from build123d import *

# Parameters (mm, degrees)
CUT_EXTRUDE1_DEPTH = 59.523499554
SKETCH3_R          = 35
SKETCH3_R_2        = 27.5
CUT_EXTRUDE2_DEPTH = 2
CUT_EXTRUDE3_START = -2
SKETCH4_R          = 35
SKETCH4_R_2        = 27.5
CUT_EXTRUDE3_DEPTH = 2
FILLET1_R          = 10
FILLET2_R          = 10


with BuildPart() as part:
    # Sketch1 → Revolve1 (revolve)
    with BuildSketch(Plane(origin=(0, 0, 0), x_dir=(0, 0, -1), z_dir=(1, 0, 0)), mode=Mode.PRIVATE) as revolve1_sk:
        Polygon((-7.5, 40), (-4.5, 40), (-2, 34), (2, 34), (4.5, 40), (7.5, 40), (7.5, 0), (-7.5, 0), align=None)
    revolve(revolve1_sk.sketch.rotate(Axis((0, 0, 652.003718611), (0, 0, -1)), 90), axis=Axis((0, 0, 652.003718611), (0, 0, -1)))

    # Sketch2 → Cut-Extrude1 (cut, through all)
    with BuildSketch(Plane.XY.offset(7.5)):
        with BuildLine():
            Line((3.2, 15.520204103), (-2.8, 15.520204103))
            Line((-2.8, 15.520204103), (-2.8, 13.71714256))
            ThreePointArc((-2.8, 13.71714256), (-0.204757333, -13.998502578), (3.2, 13.62938003))
            Line((3.2, 13.62938003), (3.2, 15.520204103))
        make_face()
    extrude(amount=-CUT_EXTRUDE1_DEPTH, mode=Mode.SUBTRACT)

    # Sketch3 → Cut-Extrude2 (cut)
    with BuildSketch(Plane.XY.offset(7.5)):
        Circle(SKETCH3_R)
        Circle(SKETCH3_R_2, mode=Mode.SUBTRACT)
    extrude(amount=-CUT_EXTRUDE2_DEPTH, mode=Mode.SUBTRACT)

    # Sketch4 → Cut-Extrude3 (cut)
    with BuildSketch(Plane(origin=(0, 0, -7.5), x_dir=(-1, 0, 0), z_dir=(0, 0, -1)).offset(CUT_EXTRUDE3_START)):
        with Locations(Location((0, 0, 0), (0, 0, 180))):
            Circle(SKETCH4_R)
        with Locations(Location((0, 0, 0), (0, 0, 180))):
            Circle(SKETCH4_R_2, mode=Mode.SUBTRACT)
    extrude(amount=CUT_EXTRUDE3_DEPTH, mode=Mode.SUBTRACT)

    # Fillet1
    # the kernel refuses this fillet: 10 mm, written as the material it adds along each edge
    with BuildSketch(Plane(origin=(0, 0, 5.5), x_dir=(1, 0, 0), z_dir=(0, -1, 0))) as fillet1_piece_1:
        with BuildLine():
            CenterArc((29, 10), FILLET1_R, 270, 36.869897646)
            Line((29, 0), (29, -0.2))
            Line((29, -0.2), (35, -0.2))
            Line((35, -0.2), (35.2, 0))
            ThreePointArc((35.2, 0), (35.2, 1), (35.12, 1.84))
            Line((35.12, 1.84), (35, 2))
        make_face()
    revolve(axis=Axis((0, 0, 5.5), (0, 0, 1)))

    # Fillet2
    # the kernel refuses this fillet: 10 mm, written as the material it adds along each edge
    with BuildSketch(Plane(origin=(0, 0, -5.5), x_dir=(1, 0, 0), z_dir=(0, 1, 0))) as fillet2_piece_1:
        with BuildLine():
            CenterArc((33.5, 10), FILLET2_R, 233.130102354, 36.869897646)
            Line((33.5, 0), (33.5, -0.2))
            Line((33.5, -0.2), (27.5, -0.2))
            Line((27.5, -0.2), (27.3, 0))
            ThreePointArc((27.3, 0), (27.3, 1), (27.38, 1.84))
            Line((27.38, 1.84), (27.5, 2))
        make_face()
    revolve(axis=Axis((0, 0, -5.5), (0, 0, -1)))


solid = part.part
For this review, take the finished solid that the model builds, in its own axes (mm). A direction names the side the tool comes from. Coordinates: 2 decimals unless noted, no trailing zeros. Loops run counter-clockwise (first coordinate to the right, second up) from the corner with the lowest first, then second, coordinate; pieces in that order, holes last. Notation, with made-up numbers: (27.25, 40.25) - (81.25, 40.25) arc R5 cw to (81.25, 49.25) - close; hole circle Ø11 at (81, 3.25). An arc over 180 degrees is marked (long way). Return JSON: item names as keys, results as strings.
Item 1: For faces 4 (the cylindrical face through (-7.587, 34.168, -6.486)), 5 (the cylindrical face through (-5.961, -26.846, 6.514)), 6 (the flat face through (-2.8, 15, 0)), 7 (the conical face through (32.708, -10.3, 2.121)), list the 3-axis set-ups (+Z, -Z, +X, -X, +Y, -Y) from which the entire face can be reached by the end or side of a thin tool; tool diameter is ignored.
Determined:
{"face 4": "-Z", "face 5": "+Z", "face 6": "+Z, -Z", "face 7": "none"}
Item 2: Insertion check: pin 1 (3 mm diameter, centred on x = 11.5, z = 4, fed in from +Y); pin 2 (8 mm diameter, centred on x = 10.5, z = 1, fed in from +Y); pin 3 (6 mm diameter, centred on y = -18.5, z = -4, fed in from +X). Each pin has a flat end and moves straight along its axis. Give the tip position at first contact, or say it passes through.
Determined:
{"pin 1": "stops at y = 38.71", "pin 2": "stops at y = 39.07", "pin 3": "stops at x = 36.86"}
Item 3: Mouldability with a two-part tool opening along X and no side actions: class faces 1 (the flat face through (-0.2, 35.4, -7.5)), 2 (the cylindrical face through (-4.43, -33.71, -0.03)), 3 (the flat face through (0, 15.52, 0)) as pulls with the +X half, pulls with the -X half, needs draft (parallel to the pull), parting line crosses it, or undercut.
Determined:
{"face 1": "needs draft", "face 2": "parting line crosses it", "face 3": "undercut"}
Item 4: For line 1 (X direction, y = 1.5, z = 6.75); line 2 (Y direction, x = 0, z = -7.1); line 3 (Y direction, x = 0, z = -0.75), list the stretches that pass through material, from the lowest coordinate up.
Determined:
{"line 1": "x = -39.97 to -33.81, -27.46 to -13.92, 13.92 to 27.46, 33.81 to 39.97", "line 2": "y = -40 to -35, -28.07 to -14, 15.52 to 28.07, 35 to 40", "line 3": "y = -34 to -14, 15.52 to 34"}
Item 5: Take a section at B-B (z = 0.25). Give the boundary of the cut face in (x, y), then the cut area to 3 significant figures.
Determined:
{"outline": "circle Ø68 at (0, 0); hole (-2.8, 13.72) arc R14 ccw (long way) to (3.2, 13.63) - (3.2, 15.52) - (-2.8, 15.52) - close", "area": "3,010 mm2"}
